from build123d import *

# Parameters (mm, degrees)
F0_R      = 32
F0_R_2    = 16
F1_DEPTH  = 38
F3_DEPTH  = 42.5
F3_FACE_R = 16
F4_DEPTH  = 56.001
F5_W      = 136
F5_H      = 44
F6_DEPTH  = 16
F7_R      = 25
F8_DEPTH  = 33


with BuildPart() as f1:
    # F0 (on Front) → F1 (new body, symmetric)
    with BuildSketch(Plane.XZ):
        Circle(F0_R)
        Circle(F0_R_2, mode=Mode.SUBTRACT)
    extrude(amount=F1_DEPTH, both=True)

    # F2 (on Top) → F3 (join, symmetric)
    with BuildSketch(Plane.XY):
        Polygon((24, 12), (0, 12), (-24, 12), (-24, -12), (24, -12), align=None)
        Polygon((0, 18), (-36, 18), (-36, -18), (36, -18), (36, 18), align=None)
        Polygon((-24, 12), (0, 12), (24, 12), (24, -12), (-24, -12), align=None, mode=Mode.SUBTRACT)
    extrude(amount=F3_DEPTH, both=True)

    # F3_face (on face) → F4 (cut, through all)
    with BuildSketch(Plane.XZ.offset(18)):
        Circle(F3_FACE_R)
    extrude(amount=-F4_DEPTH, mode=Mode.SUBTRACT)

    # F5 (on face) → F6 (join)
    with BuildSketch(Plane(origin=(0, 0, -42.5), x_dir=(1, 0, 0), z_dir=(0, 0, -1))):
        Rectangle(F5_W, F5_H)
    extrude(amount=-F6_DEPTH)

    # F7 (on Front) → F8 (cut, symmetric)
    with BuildSketch(Plane.XZ):
        Circle(F7_R)
    extrude(amount=F8_DEPTH, both=True, mode=Mode.SUBTRACT)


solid = f1.part
The listing builds one solid part. Answer for the finished solid, in the listing's coordinates (mm). A direction names the side the tool comes from. Give positions to 0.01 mm unless a question says otherwise; leave off trailing zeros. Write each loop counter-clockwise with the first axis right and the second up, starting at its lowest first coordinate (ties: lowest second). Pieces come first, ordered by that corner, then holes. Notation, with made-up numbers: (25.25, 83.5) -> (69.25, 83.5) arc R16 ccw to (69.25, 111.5) -> close; hole circle Ø7 at (-5, -9). An arc over 180 degrees is marked (long way). Use a Markdown table: item, result.
(1) Section A-A, the plane z = 0 is taken. Determine the outline of the cut face in (x, y), then the cut area to 3 significant figures.
Return value:
| item | result |
|---|---|
| outline | (-36, -18) -> (-32, -18) -> (-32, -38) -> (-16, -38) -> (-16, -33) -> (-25, -33) -> (-25, 33) -> (-16, 33) -> (-16, 38) -> (-32, 38) -> (-32, 18) -> (-36, 18) -> close; (16, -38) -> (32, -38) -> (32, -18) -> (36, -18) -> (36, 18) -> (32, 18) -> (32, 38) -> (16, 38) -> (16, 33) -> (25, 33) -> (25, -33) -> (16, -33) -> close |
| area | 1,530 mm2 |
(2) Section C-C, the plane y = -2 is taken. Determine the outline of the cut face in (x, z).
Return value:
| item | result |
|---|---|
| outline | (-68, -42.5) -> (68, -42.5) -> (68, -26.5) -> (36, -26.5) -> (36, 42.5) -> (24, 42.5) -> (24, 21.17) arc R32 ccw to (-24, 21.17) -> (-24, 42.5) -> (-36, 42.5) -> (-36, -26.5) -> (-68, -26.5) -> close; hole circle Ø50 at (0, 0); hole (-24, -26.5) -> (-17.94, -26.5) arc R32 cw to (-24, -21.17) -> close; hole (17.94, -26.5) -> (24, -26.5) -> (24, -21.17) arc R32 cw to start |
(3) Section D-D, the plane x = 20.5 is taken. Determine the outline of the cut face in (y, z), then the cut area to 3 significant figures.
Return value:
| item | result |
|---|---|
| outline | (-38, -24.57) -> (-18, -24.57) -> (-18, -26.5) -> (-22, -26.5) -> (-22, -42.5) -> (22, -42.5) -> (22, -26.5) -> (18, -26.5) -> (18, -24.57) -> (38, -24.57) -> (38, 24.57) -> (18, 24.57) -> (18, 42.5) -> (12, 42.5) -> (12, 24.57) -> (-12, 24.57) -> (-12, 42.5) -> (-18, 42.5) -> (-18, 24.57) -> (-38, 24.57) -> close; hole (-33, -14.31) -> (33, -14.31) -> (33, 14.31) -> (-33, 14.31) -> close; hole (-12, -26.5) -> (12, -26.5) -> (12, -24.57) -> (-12, -24.57) -> close |
| area | 2,790 mm2 |
(4) Find the intervals of material crossed by probe 1 along X at (y, z) = (-35, 0); probe 2 along Y at (x, z) = (23, 36); probe 3 along Y at (x, z) = (16.5, 0.5), in increasing order. Write a range as from..to.
Return value:
| item | result |
|---|---|
| probe 1 | -32..-16, 16..32 |
| probe 2 | -18..-12, 12..18 |
| probe 3 | -38..-33, 33..38 |
(5) Determine the mould class of faces 6 (the flat face through (-15, 38, -7)), 7 (the flat face through (-0.3, 33, -16.3)), 8 (the cylindrical face through (-4.166, -28.14, 31.728)) for opening direction X: released by +X, released by -X, zero draft, split by the parting line, or undercut.
Return value:
| item | result |
|---|---|
| face 6 | zero draft |
| face 7 | undercut |
| face 8 | split by the parting line |
(6) Section B-B, the plane x = 0 is taken. Determine the outline of the cut face in (y, z).
Return value:
| item | result |
|---|---|
| outline | (-38, -32) -> (-22, -32) -> (-22, -42.5) -> (22, -42.5) -> (22, -32) -> (38, -32) -> (38, -16) -> (33, -16) -> (33, -25) -> (-33, -25) -> (-33, -16) -> (-38, -16) -> close; (-38, 16) -> (-33, 16) -> (-33, 25) -> (33, 25) -> (33, 16) -> (38, 16) -> (38, 32) -> (18, 32) -> (18, 42.5) -> (12, 42.5) -> (12, 32) -> (-12, 32) -> (-12, 42.5) -> (-18, 42.5) -> (-18, 32) -> (-38, 32) -> close |
(7) For faces 1 (the flat face through (-24, 0, 32)), 2 (the flat face through (36, 0, 8)), 3 (the flat face through (-1, 0, -42.5)), 4 (the cylindrical face through (23.846, -0.462, 7.509)), 5 (the flat face through (68, 0, -35)), determine the directions among +Z, -Z, +X, -X, +Y, -Y from which every point of the face is accessible in a straight line to the end or side of a thin tool.
Return value:
| item | result |
|---|---|
| face 1 | +Z |
| face 2 | +Z, +X, +Y, -Y |
| face 3 | -Z, +X, -X, +Y, -Y |
| face 4 | none |
| face 5 | +Z, -Z, +X, +Y, -Y |
(8) Flat-ended cylindrical pins translate along their axes: P1, Ø2, axis at x = -7.5, z = -33, coming from the +Y side; P2, Ø6.5, axis at y = -0.5, z = 28.5, coming from the +X side; P3, Ø5, axis at x = -22.5, z = -35.5, coming from the -Y side. Find the tip coordinate at first contact, or state that the pin passes through.
Return value:
| item | result |
|---|---|
| P1 | y = 22 |
| P2 | x = 36 |
| P3 | y = -22 |
